Verification items for the finished model (mm, model axes). Face numbers are marked on the shaded views. A direction names the side the tool comes from. Give positions to 0.01 mm unless a question says otherwise; leave off trailing zeros. Loops run counter-clockwise (first coordinate to the right, second up) from the corner with the lowest first, then second, coordinate; pieces in that order, holes last. Notation, with made-up numbers: (13.25, 46) - (58.25, 46) arc R17 ccw to (58.25, 60) - close; hole circle Ø7 at (4, 16.25). An arc over 180 degrees is marked (long way). One line per item, written item: value. Start each with the question number.
1. Sectioned sample at B-B (z = 15). Record the cut outline in (x, y).
2. Scan lines: L1, parallel to Y at x = 28, z = 11; L2, parallel to Y at x = 4.5, z = 25; L3, parallel to Z at x = 0, y = 7.5. Record each from-to range of solid material in increasing order. Write a range as [from, to].
3. Sectioned sample at A-A (x = 0). Record the cut outline in (y, z) (3 decimals), plus the area to 3 significant figures.
4. Gauge pin test, flat ends, axial feed: pin 1 (9 mm diameter, centred on y = 0, z = 35.5, fed in from -X); pin 2 (2 mm diameter, centred on y = 2.5, z = 16.5, fed in from +X); pin 3 (5 mm diameter, centred on x = -4, y = -4, fed in from -Z). Record the tip position at first contact, or that the pin passes through.
5. Mould release check, pull along Y, two halves, no side actions. Record for the marked faces 4, 5 and 6: pulls with the +Y half, pulls with the -Y half, needs draft (parallel to the pull), parting line crosses it, or undercut.
6. Sectioned sample at C-C (y = 6.75). Record the cut outline in (x, z).
7. Access from +Z, -Z, +X, -X, +Y, -Y to the whole of each face (thin tool, end or side, straight path). Record for the marked faces 1, 2 and 3.
8. Sectioned sample at D-D (z = 25). Record the cut outline in (x, y), plus the area to 3 significant figures.
from build123d import *

# Parameters (mm, degrees)
F1_DEPTH       = 9.5
F3_D           = 6.8
F3_START       = 2
F3_CSINK_D     = 8.5
F3_CSINK_ANGLE = 90
F5_D           = 10.25
F5_START       = 22.0000001
F5_CBORE_D     = 16
F5_CBORE_DEPTH = 10.5
F6_W           = 29.5
F6_H           = 4
F7_DEPTH       = 19
F8_R           = 6
F9_R           = 6


with BuildPart() as f1:
    # F0 (on Front) → F1 (new body, symmetric)
    with BuildSketch(Plane.XZ):
        with BuildLine():
            Line((-34.5, 2), (-21.9089023002, 2))
            ThreePointArc((-21.9089023002, 2), (-14.8323969742, 16.2480768093), (0, 22))
            ThreePointArc((0, 22), (14.8323969742, 16.2480768093), (21.9089023002, 2))
            Line((21.9089023002, 2), (34.5, 2))
            Line((34.5, 2), (34.5, 15))
            Line((34.5, 15), (17, 28))
            Line((17, 28), (17, 46))
            Line((17, 46), (0, 46))
            Line((0, 46), (-17, 46))
            Line((-17, 46), (-17, 28))
            Line((-17, 28), (-34.5, 15))
            Line((-34.5, 15), (-34.5, 2))
        make_face()
    extrude(amount=F1_DEPTH, both=True)

    # F3 (through all)
    # its depths count from where the whole tool has entered the part; down to there all is cleared
    with Locations(Plane(origin=(0, 0, 0), x_dir=(1, 0, 0), z_dir=(0, 0, -1)).offset(-F3_START)):
        with Locations((28, 0), (-28, 0)):
            CounterSinkHole(F3_D / 2, F3_CSINK_D / 2, counter_sink_angle=F3_CSINK_ANGLE)

    # F5 (through all)
    # its depths count from where the whole tool has entered the part; down to there all is cleared
    with Locations(Plane(origin=(0, 0, 0), x_dir=(1, 0, 0), z_dir=(0, 0, -1)).offset(-F5_START)):
        with Locations((0, 0)):
            CounterBoreHole(F5_D / 2, F5_CBORE_D / 2, F5_CBORE_DEPTH)

    # F6 (on face) → F7 (cut)
    with BuildSketch(Plane.XZ.offset(9.5)):
        with Locations((-2.25, 44)):
            Rectangle(F6_W, F6_H)
    extrude(amount=-F7_DEPTH, mode=Mode.SUBTRACT)

    # F8
    f8_edges = [f1.edges().sort_by_distance(p)[0] for p in [
        (17, 0, 28),
        (-17, 0, 28),
    ]]
    fillet(f8_edges, radius=F8_R)

    # F9
    f9_edges = [f1.edges().sort_by_distance(p)[0] for p in [
        (34.5, 0, 15),
        (-34.5, 0, 15),
    ]]
    fillet(f9_edges, radius=F9_R)


solid = f1.part
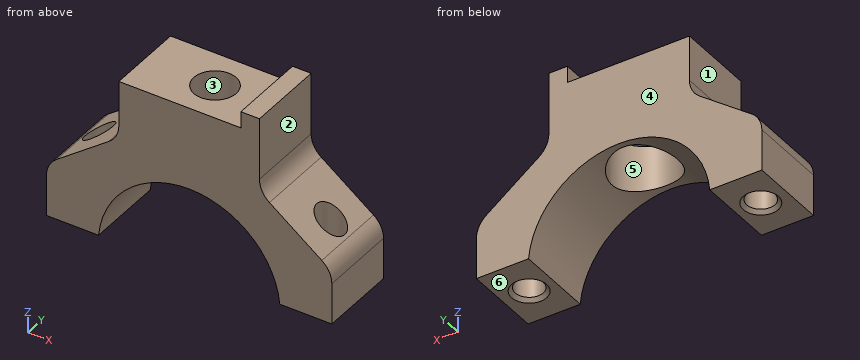
Results are:
1. outline: (-33.69, -9.5) - (-16.09, -9.5) - (-16.09, 9.5) - (-33.69, 9.5) - close; (16.09, -9.5) - (33.69, -9.5) - (33.69, 9.5) - (16.09, 9.5) - close; hole circle Ø6.8 at (-28, 0); hole circle Ø6.8 at (28, 0)
2. L1: y = [-9.5, -3.4], [3.4, 9.5]
2. L2: y = [-9.5, -6.61], [6.61, 9.5]
2. L3: z = [32.5, 42]
3. outline: (-9.5, 22) - (-8, 22) - (-8, 32.5) - (-5.125, 32.5) - (-5.125, 42) - (-9.5, 42) - close; (5.125, 32.5) - (8, 32.5) - (8, 22) - (9.5, 22) - (9.5, 42) - (5.125, 42) - close
3. area: 115 mm^2
4. pin 1: stops at x = -17
4. pin 2: stops at x = 33.36
4. pin 3: stops at z = 21.07
5. face 4: pulls with the +Y half
5. face 5: undercut
5. face 6: needs draft
6. outline: (-34.5, 2) - (-21.91, 2) arc R22 cw to (-4.29, 21.58) - (-4.29, 32.5) - (4.29, 32.5) - (4.29, 21.58) arc R22 cw to (21.91, 2) - (34.5, 2) - (34.5, 11.98) arc R6 ccw to (32.08, 16.8) - (19.42, 26.2) arc R6 cw to (17, 31.02) - (17, 46) - (12.5, 46) - (12.5, 42) - (-17, 42) - (-17, 31.02) arc R6 cw to (-19.42, 26.2) - (-32.08, 16.8) arc R6 ccw to (-34.5, 11.98) - close
7. face 1: +Z, -X, +Y, -Y
7. face 2: +Z, +X, +Y, -Y
7. face 3: +Z, -Z
8. outline: (-21.04, -9.5) - (21.04, -9.5) - (21.04, 9.5) - (-21.04, 9.5) - close; hole circle Ø16 at (0, 0)
8. area: 598 mm^2
